Can you work these out from the model? Positions are in its coordinate system, mm. A direction names the side the tool comes from. Give positions to 0.01 mm unless a question says otherwise; leave off trailing zeros. Write each loop counter-clockwise with the first axis right and the second up, starting at its lowest first coordinate (ties: lowest second). Pieces come first, ordered by that corner, then holes.
```python
from build123d import *

# Parameters (mm, degrees)
STOCK_ACRYLIC_PARTS_1_OUTLINE_R = 1
STOCK_ACRYLIC_PARTS_1_DEPTH     = 3
SKETCH2_W                       = 1.1125911
SKETCH2_H                       = 0.19748244
CUT_EXTRUDE1_DEPTH              = 963.439452829


# Read off the part's stored shape, not the designer's step: Stock-acrylic parts-1
with BuildPart() as part:
    # Stock-acrylic parts-1 outline → Stock-acrylic parts-1 (new body)
    with BuildSketch(Plane.XY):
        with BuildLine():
            Line((832.672571413, 113.966353753), (830.641097077, 110.901419151))
            ThreePointArc((830.641097077, 110.901419151), (830.000519222, 106.767582069), (832.725500034, 103.593715565))
            ThreePointArc((832.725500034, 103.593715565), (862.032980753, 94.202742704), (892.672186774, 91.311747764))
            ThreePointArc((892.672186774, 91.311747764), (923.311281331, 94.203923771), (952.618400028, 103.596026361))
            ThreePointArc((952.618400028, 103.596026361), (955.343258494, 106.769997904), (954.702521289, 110.90381029))
            Line((954.702521289, 110.90381029), (952.670928809, 113.968666581))
            ThreePointArc((952.670928809, 113.968666581), (950.188269571, 114.970742443), (947.519688189, 114.755274729))
            Line((947.519688189, 114.755274729), (932.172066536, 111.200676976))
            ThreePointArc((932.172066536, 111.200676976), (931.366268377, 111.218620275), (930.686084525, 111.65103508))
            ThreePointArc((930.686084525, 111.65103508), (930.167968592, 111.983103753), (929.557642996, 112.061947844))
            ThreePointArc((929.557642996, 112.061947844), (892.663576086, 110.941819466), (855.769509176, 112.061947844))
            ThreePointArc((855.769509176, 112.061947844), (855.167872493, 111.978815429), (854.65750502, 111.649569718))
            ThreePointArc((854.65750502, 111.649569718), (853.977337838, 111.217128694), (853.171540371, 111.199154333))
            Line((853.171540371, 111.199154333), (837.823781708, 114.753160468))
            ThreePointArc((837.823781708, 114.753160468), (835.155192022, 114.968525315), (832.672571413, 113.966353753))
        make_face()
        with Locations((862.668334441, 102.956811364)):
            Circle(STOCK_ACRYLIC_PARTS_1_OUTLINE_R, mode=Mode.SUBTRACT)
        Polygon((891.782840588, 107.202653527), (892.63595645, 107.317748247), (893.489072311, 107.202653527), (894.309403409, 106.861792394), (895.065424878, 106.308263949), (895.728083238, 105.56333998), (896.2719129, 104.655647498), (896.676014794, 103.620068616), (896.924859512, 102.496400048), (897.00888409, 101.327823749), (896.924859512, 100.15924745), (896.676014794, 99.035578883), (896.2719129, 98), (895.728083238, 97.092307518), (895.065424878, 96.347383549), (894.309403409, 95.793855104), (893.489072311, 95.452993971), (892.63595645, 95.337899251), (891.782840588, 95.452993971), (890.962509491, 95.793855104), (890.206488022, 96.347383549), (889.543829662, 97.092307518), (889, 98), (888.595898106, 99.035578883), (888.347053388, 100.15924745), (888.263028809, 101.327823749), (888.347053388, 102.496400048), (888.595898106, 103.620068616), (889, 104.655647498), (889.543829662, 105.56333998), (890.206488022, 106.308263949), (890.962509491, 106.861792394), align=None, mode=Mode.SUBTRACT)
        with Locations((922.675390412, 102.956811364)):
            Circle(STOCK_ACRYLIC_PARTS_1_OUTLINE_R, mode=Mode.SUBTRACT)
    extrude(amount=STOCK_ACRYLIC_PARTS_1_DEPTH)

    # Sketch2 → Cut-Extrude1 (cut, through all)
    with BuildSketch(Plane.XY.offset(3)):
        with Locations((892.663576086, 111.040560686)):
            Rectangle(SKETCH2_W, SKETCH2_H)
    extrude(amount=-CUT_EXTRUDE1_DEPTH, mode=Mode.SUBTRACT)


solid = part.part
```
1) Suppose I cut it at C-C on x = 869. Write out the boundary of the cut face in (y, z), plus the area to 3 significant figures.
Values follow:
outline: (92.95, 0) - (111.4, 0) - (111.4, 3) - (92.95, 3) - close
area: 55.3 mm2
2) For pin 1 Ø1.5 at (x, z) = (856, 0.5) entering from +Y; pin 2 Ø0.6 at (x, z) = (892.5, 2) entering from +Y; pin 3 Ø1 at (x, z) = (848, 2) entering from +Y, each with a flat end and sliding along its axis, tell me the tip position at first contact or that it passes through.
Values follow:
pin 1: stops at y = 112.07
pin 2: stops at y = 110.94
pin 3: stops at y = 112.51
3) Suppose I cut it at B-B on x = 906. Write out the boundary of the cut face in (y, z).
Values follow:
outline: (91.75, 0) - (111.09, 0) - (111.09, 3) - (91.75, 3) - close
4) For faces 1 (the face through (863.62, 103.26, 1.48)), 2 (the face through (939.953, 113.003, 1.479)), which set-ups out of +Z, -Z, +X, -X, +Y, -Y let a thin tool reach every point of the face, with its end or its side?
Values follow:
face 1: +Z, -Z
face 2: +Z, -Z, +Y
5) If we mould it in two halves opening along Y, with no side actions, what happens to faces 3 (the face through (923.63, 103.26, 1.48)), 4 (the face through (892, 109, 3)), 5 (the face through (911.65, 111.24, 1.48))? For each: +Y half, -Y half, draft (parallel to the pull), parting line (faces both ways), or undercut.
Values follow:
face 3: undercut
face 4: draft
face 5: +Y half
6) Please list where these lines run through material, in increasing order: L1, parallel to X at y = 102.25, z = 2.4; L2, parallel to Y at x = 891, z = 2.8; L3, parallel to Y at x = 893.5, z = 2.05.
Values follow:
L1: x = 835.85 to 861.96, 863.38 to 888.33, 896.94 to 921.97, 923.38 to 949.49
L2: y = 91.3 to 95.78, 106.88 to 110.94
L3: y = 91.3 to 95.46, 107.2 to 110.94
7) Suppose I cut it at A-A on z = 2.35. State how many separate pieces and enclosed holes the cut face has, plus the area to 3 significant figures.
Values follow:
separate pieces: 1
enclosed holes: 3
area: 1,970 mm2
